Design review of the part built by this model. Coordinates are the model's own, in mm. A direction names the side the tool comes from. Coordinates: 2 decimals unless noted, no trailing zeros. Loops run counter-clockwise (first coordinate to the right, second up) from the corner with the lowest first, then second, coordinate; pieces in that order, holes last. Notation, with made-up numbers: M 25,86 L 84,86 A9 ccw 84,94 Z; hole C 56.25,57 d6. An arc over 180 degrees is marked long. Put each result on its own line as item: value. Start each with the question number.
(1) For probe 1 along Z at (x, y) = (0, -2); probe 2 along Y at (x, z) = (-16.5, 9) (3 decimals); probe 3 along Z at (x, y) = (0, 0.25), list the stretches that pass through material, from the lowest coordinate up. Write a range as [from, to].
(2) Take a section at A-A, the plane z = 0. Give the boundary of the cut face in (x, y) (3 decimals).
(3) For faces 4 (the flat face through (0, 0, 17)), 5 (the conical face through (-12.29, -3.68, -3.87)), list the 3-axis set-ups (+Z, -Z, +X, -X, +Y, -Y) from which the entire face can be reached by the end or side of a thin tool; tool diameter is ignored.
(4) Take a section at B-B, the plane x = 0. Give the boundary of the cut face in (y, z) (3 decimals).
(5) Take a section at C-C, the plane y = 1.25. Give the boundary of the cut face in (x, z), then the cut area to 3 significant figures.
(6) Take a section at D-D, the plane y = 4.75. Give the boundary of the cut face in (x, z) (3 decimals).
(7) Clearance check with flat-ended pins moving along their axes: pin 1 (10 mm diameter, centred on x = -7.5, y = -4, fed in from -Z); pin 2 (1 mm diameter, centred on x = -10, y = -2, fed in from -Z); pin 3 (8 mm diameter, centred on x = 13, z = 1, fed in from +Y); pin 4 (10 mm diameter, centred on x = 3, z = -0.5, fed in from +Y). State where each tip first meets the part, or that it passes through.
(8) The part is to be moulded in two halves that separate along Z. For faces 1 (the cylindrical face through (4.13, 4.32, 18.597)), 2 (the flat face through (6, -13.643, -16)), 3 (the cylindrical face through (-5.86, 0.044, 11.267)), say which applies: +Z half, -Z half, draft (parallel to the pull), parting line (faces both ways), or undercut.
```python
from build123d import *

# Parameters (mm, degrees)
FILLET3_R = 0.762


with BuildPart() as part:
    # Sketch1 → Revolve1 (revolve)
    with BuildSketch(Plane.XY, mode=Mode.PRIVATE) as revolve1_sk:
        Polygon((12.7, -3.175), (12.7, 3.175), (18.288, 8.763), (19.05, 8.763), (19.05, 0), (16.764, 0), (16.764, -3.175), (19.05, -3.175), (19.05, -13.642888968), (16.51, -13.642888968), align=None)
    revolve(revolve1_sk.sketch.rotate(Axis((0, 44.779079664, 0), (0, -1, 0)), 180), axis=Axis((0, 44.779079664, 0), (0, -1, 0)))

    # Fillet3
    fillet3_edges = [part.edges().sort_by_distance(p)[0] for p in [
        (18.288, 8.763, 0),
    ]]
    fillet(fillet3_edges, radius=FILLET3_R)


solid = part.part
```
Computed values:
1. probe 1: z = [-16.76, -12.7], [12.7, 16.76]
1. probe 2: y = [-13.643, -3.175], [0, 8.763]
1. probe 3: z = [-19.05, -12.7], [12.7, 19.05]
2. outline: M -19.05,-13.643 L -16.51,-13.643 L -12.7,-3.175 L -12.7,3.175 L -18.065,8.54 A0.762 ccw -18.604,8.763 L -19.05,8.763 L -19.05,0 L -16.764,0 L -16.764,-3.175 L -19.05,-3.175 Z; M 12.7,-3.175 L 16.51,-13.643 L 19.05,-13.643 L 19.05,-3.175 L 16.764,-3.175 L 16.764,0 L 19.05,0 L 19.05,8.763 L 18.604,8.763 A0.762 ccw 18.065,8.54 L 12.7,3.175 Z
3. face 4: none
3. face 5: -Y
4. outline: M -13.643,-19.05 L -3.175,-19.05 L -3.175,-16.764 L 0,-16.764 L 0,-19.05 L 8.763,-19.05 L 8.763,-18.604 A0.762 ccw 8.54,-18.065 L 3.175,-12.7 L -3.175,-12.7 L -13.643,-16.51 Z; M -13.643,16.51 L -3.175,12.7 L 3.175,12.7 L 8.54,18.065 A0.762 ccw 8.763,18.604 L 8.763,19.05 L 0,19.05 L 0,16.764 L -3.175,16.764 L -3.175,19.05 L -13.643,19.05 Z
5. outline: C 0,0 d38.1; hole C 0,0 d25.4
5. area: 633 mm^2
6. outline: C 0,0 d38.1; hole C 0,0 d28.55
7. pin 1: stops at z = -18.89
7. pin 2: stops at z = -13.81
7. pin 3: stops at y = 7.51
7. pin 4: passes through
8. face 1: parting line
8. face 2: draft
8. face 3: undercut
